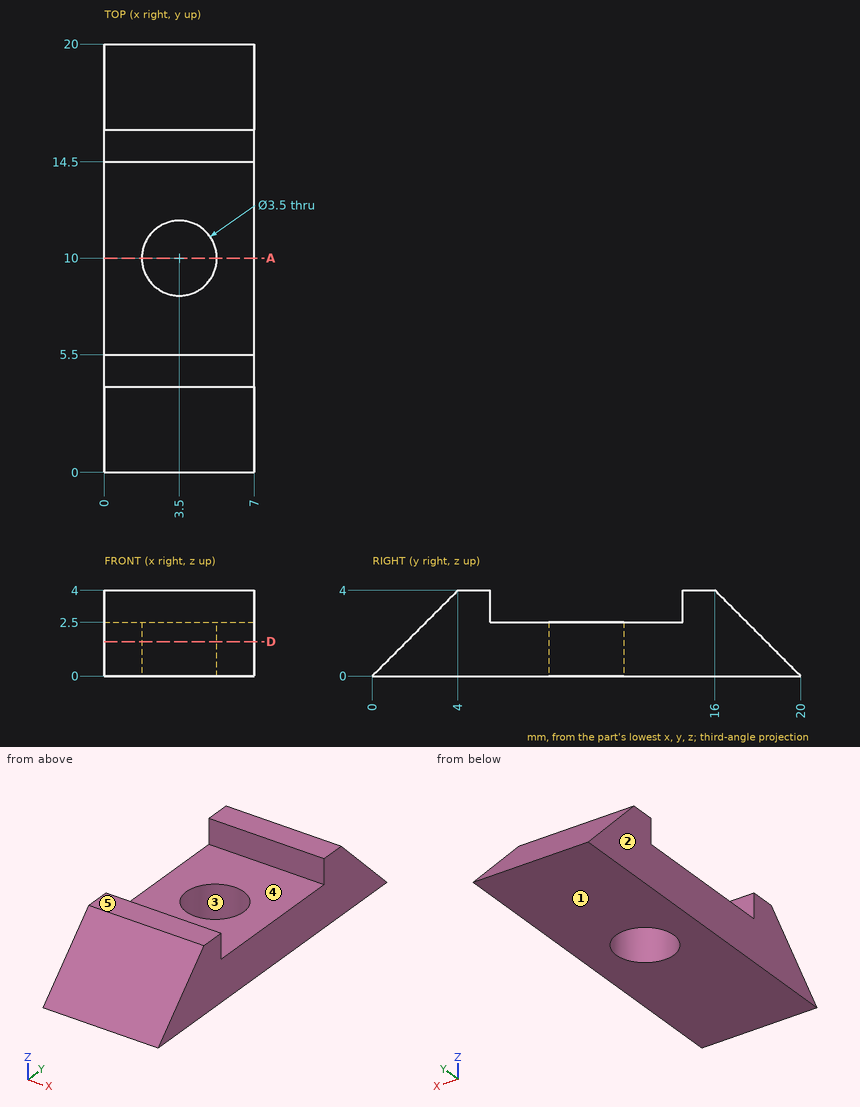
Verification items for this drawing (mm, ordinates from the low corner). A direction names the side the tool comes from. Give positions to 0.01 mm unless a question says otherwise; leave off trailing zeros. Loops run counter-clockwise (first coordinate to the right, second up) from the corner with the lowest first, then second, coordinate; pieces in that order, holes last. Notation, with made-up numbers: M 38,54.25 L 82,54.25 A17 ccw 82,64.25 Z; hole C -27.75,-5 d1. An arc over 180 degrees is marked long. Answer as a JSON object with one key per item and string values. Group by question number.
Item 1: Gauge pin test, flat ends, axial feed: pin 1 (2 mm diameter, centred on y = 14.5, z = 1.5, fed in from -X); pin 2 (1.5 mm diameter, centred on x = 5.5, z = 1, fed in from +Y); pin 3 (0.8 mm diameter, centred on x = 4, z = 3.5, fed in from -Y); pin 4 (2 mm diameter, centred on x = 1, z = 2.5, fed in from +Y). Record the tip position at first contact, or that the pin passes through.
Item 2: Access from +Z, -Z, +X, -X, +Y, -Y to the whole of each face (thin tool, end or side, straight path). Record for the marked faces 4 and 5.
Item 3: Sectioned sample at D-D on z = 1.6. Record the boundary of the cut face in (x, y).
Item 4: Mould release check, pull along X, two halves, no side actions. Record for the marked faces 1, 2 and 3: pulls with the +X half, pulls with the -X half, needs draft (parallel to the pull), parting line crosses it, or undercut.
Item 5: Material ranges on L1, parallel to Z at x = 5.25, y = 2.5; L2, parallel to Y at x = 3.5, z = 1.95; L3, parallel to Y at x = 3.5, z = 1, recorded low to high.
Item 6: Sectioned sample at A-A on y = 10. Record the boundary of the cut face in (x, z), plus the area to 3 significant figures.
Findings below:
{
 "1": {"pin 1": "x = 0", "pin 2": "y = 19.75", "pin 3": "y = 3.1", "pin 4": "y = 18.5"},
 "2": {"face 4": "+Z, +X, -X", "face 5": "+Z, +X, -X, +Y, -Y"},
 "3": {"outline": "M 0,1.6 L 7,1.6 L 7,18.4 L 0,18.4 Z; hole C 3.5,10 d3.5"},
 "4": {"face 1": "needs draft", "face 2": "pulls with the -X half", "face 3": "undercut"},
 "5": {"L1": "0 to 2.5", "L2": "1.95 to 8.25, 11.75 to 18.05", "L3": "1 to 8.25, 11.75 to 19"},
 "6": {"outline": "M 0,0 L 1.75,0 L 1.75,2.5 L 0,2.5 Z; M 5.25,0 L 7,0 L 7,2.5 L 5.25,2.5 Z", "area": "8.75 mm2"}
}
